Autodesk Inventor part; units mm, degrees
ref_plane "YZ Plane" through (0, 0, 0) normal (1, 0, 0) x (0, 1, 0)
ref_plane "XZ Plane" through (0, 0, 0) normal (0, 1, 0) x (-1, 0, 0)
ref_plane "XY Plane" through (0, 0, 0) normal (0, 0, 1) x (1, 0, 0)
sketch "Sketch1" plane through (0, 0, 0) normal (0, 1, 0) x (-1, 0, 0)
  line L0 (10, -17.5) -> (-10, -17.5)
  line L1 (-10, -17.5) -> (-10, 18.5)
  line L2 (-10, 18.5) -> (10, 18.5)
  line L3 (10, 18.5) -> (10, -17.5)
  point P0 (0, 0)
  dimension "d0" = 20
  dimension "d1" = 36
  dimension "d2" = 17.5
  dimension "d3" = 10
extrude "Plate1" add sketch "Sketch1" along normal blind 1.5
sketch "Sketch2" plane through (-10, 0, -19) normal (0, 0, 1) x (1, 0, 0)
  line L0 (20, 0) -> (0, 0)
  line L1 (0, 0) -> (0, 45.1)
  line L2 (0, 45.1) -> (20, 45.1)
  line L3 (20, 45.1) -> (20, 0)
edge flange "Flange1" height 45.1 angle 90 thickness 1.5 bend radius 0.31 thickness toward (0, 0, 1) relief tear relief width 1.5 relief depth 0.75 edges at (0, 1.5, -17.5) wall of the first edge with corners at (10, 0, -19) (-10, 0, -19) (-10, 45.1, -19) (10, 45.1, -19)
bend "Bend1"
corner "Corner1"
sketch "Sketch3" plane through (10, 0, 20) normal (0, 0, -1) x (-1, 0, 0)
  line L0 (20, 0) -> (0, 0)
  line L1 (0, 0) -> (0, 45.1)
  line L2 (0, 45.1) -> (20, 45.1)
  line L3 (20, 45.1) -> (20, 0)
edge flange "Flange2" height 45.1 angle 90 thickness 1.5 bend radius 0.31 thickness toward (0, 0, -1) relief tear relief width 1.5 relief depth 0.75 edges at (0, 1.5, 18.5) wall of the first edge with corners at (-10, 0, 20) (10, 0, 20) (10, 45.1, 20) (-10, 45.1, 20)
bend "Bend2"
corner "Corner2"
sketch "Sketch4" plane through (-10, 45.1, 20) normal (0, 0, 1) x (1, 0, 0)
  circle A0 centre (10, -10) radius 10
  line L0 (0, 0) -> (20, 0)
  line L1 (0, 0) -> (20, 0)
  line L2 (20, 0) -> (20, -10)
  line L3 (20, -10) -> (0, -10)
  line L4 (0, -10) -> (0, 0)
  line L5 (0, -43.29) -> (0, 0)
  point P0 (10, -45.1)
  point P1 (10, -10)
  point P2 (20, 0)
  point P3 (10, 0)
  point P4 (0, -10)
  point P5 (8.5893, 0)
  point P6 (0, -10)
  dimension "d26" = 20
  dimension "d25" = 10
  dimension "d27" = 10
  dimension "d28" = 10
extrude "Extrusion1" cut sketch "Sketch4" against normal blind 10 contours L4 L0 A0 | A0 L0 L2
sketch "Sketch5" plane through (10, 45.1, -19) normal (0, 0, -1) x (-1, 0, 0)
  arc A0 (20, -10) -> (0, -10) centre (10, -10) ccw
  point P0 (10, -45.1)
hole "Hole1" at (0, 35.1, -19) direction (0, 0, 1) diameter 13.5 depth 1.5
sketch "Sketch6" plane through (10, 45.1, -19) normal (0, 0, -1) x (-1, 0, 0)
  circle A0 centre (10, -10) radius 6.75
  line L0 (0, 0) -> (20, 0)
  line L1 (0, -43.29) -> (0, 0)
  line L2 (24, 0) -> (-4, 0)
  line L3 (-4, 0) -> (-4, -9.9)
  line L4 (-4, -9.9) -> (24, -9.9)
  line L5 (24, -9.9) -> (24, 0)
  point P0 (10, -45.1)
  point P1 (20, 0)
  point P2 (6.005, 0)
  point P3 (13.995, 0)
  dimension "d38" = 9.9
  dimension "d39" = 4
  dimension "d40" = 28
extrude "Extrusion2" cut sketch "Sketch6" against normal blind 10 contours L4 A0 | A0 L4 L1 L0 L2 L5 | L4 L3 L2 L1 picked at (7.8223, -9.3675)
fillet "Fillet1" radius 1 2 edges at (-10, 35.2, -18.25) (10, 35.2, -18.25)
sketch "Sketch7" plane through (-10, 1.81, 20) normal (0, 0, 1) x (1, 0, 0)
  arc A0 (20, 33.29) -> (0, 33.29) centre (10, 33.29) ccw
  point P0 (10, -1.81)
hole "Hole2" at (0, 35.1, 20) direction (0, 0, -1) diameter 5.1 depth 1.5
sketch "Sketch8" plane through (0, 0, 0) normal (0, -1, 0) x (1, 0, 0)
  line L0 (2.55, 18.5) -> (-2.55, 18.5)
  line L1 (-10, 18.5) -> (10, 18.5)
  line L2 (10, 18.5) -> (-10, 18.5)
  line L3 (10, 18.19) -> (-10, 18.19)
  line L4 (-10, -17.19) -> (-10, 18.19)
  line L5 (-10, -17.19) -> (10, -17.19)
  line L6 (10, 18.19) -> (10, -17.19)
  point P0 (0, 0)
  point P1 (7, 9.5)
  point P2 (7, -4.5)
  point P3 (-7, 9.5)
  point P4 (-7, -4.5)
  dimension "d51" = 9
  dimension "d52" = 3
  dimension "d55" = 14
  dimension "d58" = 14
hole "Hole3" at (7, 0, 9.5) at (7, 0, -4.5) at (-7, 0, 9.5) at (-7, 0, -4.5) direction (0, 1, 0) diameter 3 depth 1.5
sketch "Sketch11" plane through (-10, 1.81, -17.5) normal (0, 0, 1) x (1, 0, 0)
  circle A0 centre (18, 26.39) radius 0.7835
  circle A1 centre (2, 26.39) radius 0.7835
  circle A2 centre (17, 13.17) radius 0.7835
  circle A3 centre (3, 13.17) radius 0.7835
  circle A4 centre (10, 5.87) radius 0.7835
  point P0 (10, -1.81)
hole "Hole6" at (-8, 28.2, -17.5) at (-7, 14.98, -17.5) at (0, 7.68, -17.5) at (7, 14.98, -17.5) at (8, 28.2, -17.5) direction (0, 0, -1) diameter 2.1 depth 1.5
sketch "Sketch12" plane through (-10, 1.81, 20) normal (0, 0, 1) x (1, 0, 0)
  line L0 (20, -1.81) -> (0, -1.81)
  circle A0 centre (10, 5.87) radius 1.05
  point P0 (10, -1.81)
hole "Hole7" at (0, 7.68, 20) direction (0, 0, -1) diameter 3 depth 1.5
equation "\"d36\" = Thickness"
equation "\"d49\" = Thickness"
equation "\"d66\" = Thickness"
equation "\"d87\" = Thickness"
equation "\"d94\" = Thickness"
equation "\"d4\" = Thickness"
equation "\"d5\" = BendReliefWidth"
equation "\"d6\" = BendReliefDepth"
equation "\"d7\" = MinimumRemnant"
equation "\"d8\" = TransitionRadius"
equation "\"d11\" = BendRadius"
equation "\"d12\" = CornerReliefSize"
equation "\"d13\" = GapSize"
equation "\"d14\" = JacobiRadiusSize"
equation "\"d15\" = BendReliefWidth"
equation "\"d16\" = BendReliefDepth"
equation "\"d17\" = MinimumRemnant"
equation "\"d18\" = TransitionRadius"
equation "\"d21\" = BendRadius"
equation "\"d22\" = CornerReliefSize"
equation "\"d23\" = GapSize"
equation "\"d24\" = JacobiRadiusSize"
equation "\"BendReliefWidth\" = Thickness"
equation "\"BendReliefDepth\" = 0.5 * Thickness"
equation "\"CornerReliefSize\" = 4 * Thickness"
equation "\"MinimumRemnant\" = 2 * Thickness"
equation "\"TransitionRadius\" = BendRadius"
equation "\"JacobiRadiusSize\" = BendRadius"
equation "\"GapSize\" = Thickness"
properties part number "axis_9_bottom_frame" material "Aluminum 6061-AHC"
CAD build for the part. Positions are in the model's coordinates, mm. A direction names the side the tool comes from. Round coordinates to 2 decimals unless told otherwise and drop trailing zeros. Write each loop counter-clockwise with the first axis right and the second up, starting at its lowest first coordinate (ties: lowest second). Pieces come first, ordered by that corner, then holes.
(1) Probe line 1 along X through (y, z) = (1.05, 9.5); line 2 along Z through (x, y) = (6, 28.5); line 3 along X through (y, z) = (28, -18). List the from-to ranges inside material, lowest first.
(2) Drop flat-ended pins along their axis: P1, Ø5, axis at x = 7, z = -4.5, coming from the +Y side; P2, Ø2.5, axis at x = -8, y = 28.2, coming from the -Z side; P3, Ø2.5, axis at x = 0, y = 7.68, coming from the +Z side; P4, Ø1.6, axis at x = -7.5, z = -18, coming from the +Y side. Give the stop position or say it passes through.
(3) Slice it at A-A, the plane y = 25.5. Write the cut outline in (x, z).
(4) 3-axis set-ups, long thin cutter, end or side, ignore diameter. For faces 1 (the face through (9.699, 34.915, -18.26)), 2 (the face through (0, 1.5, 1)), 3 (the face through (-9.715, 34.899, -18.26)), 4 (the face through (-7.32, 13.98, -18.26)): which of +Z, -Z, +X, -X, +Y, -Y reach the whole face in a straight line?
(5) Mould opens along Y. For faces 5 (the face through (-0.07, 9.18, 19.24)), 6 (the face through (-8.71, 28.974, -18.26)), 7 (the face through (10, 1, 1)), 8 (the face through (0.2, 45.1, 19.3)) say: pulls with the +Y half, pulls with the -Y half, needs draft (parallel to the pull), parting line crosses it, or undercut.
(6) Slice it at C-C, the plane y = 7.68. Write the cut outline in (x, z), and give its area (4 significant figures).
(7) Slice it at D-D, the plane y = 14.98. Write the cut outline in (x, z), and give its area (3 significant figures).
(8) Slice it at B-B, the plane z = 9.5. Write the cut outline in (x, y).
From the geometry:
1. line 1: x = -10 to -8.5, -5.5 to 5.5, 8.5 to 10
1. line 2: z = -19 to -17.5, 18.5 to 20
1. line 3: x = -10 to -9.03, -6.97 to 6.97, 9.03 to 10
2. P1: stops at y = 1.5
2. P2: stops at z = -19
2. P3: stops at z = -17.5
2. P4: stops at y = 35.2
3. outline: (-10, -19) - (10, -19) - (10, -17.5) - (-10, -17.5) - close; (-10, 18.5) - (10, 18.5) - (10, 20) - (-10, 20) - close
4. face 1: -Z, +X, +Y
4. face 2: +X, -X, +Y
4. face 3: -Z, -X, +Y
4. face 4: -Z
5. face 5: undercut
5. face 6: undercut
5. face 7: needs draft
5. face 8: pulls with the +Y half
6. outline: (-10, -19) - (-1.05, -19) - (-1.05, -17.5) - (-10, -17.5) - close; (-10, 18.5) - (-1.5, 18.5) - (-1.5, 20) - (-10, 20) - close; (1.05, -19) - (10, -19) - (10, -17.5) - (1.05, -17.5) - close; (1.5, 18.5) - (10, 18.5) - (10, 20) - (1.5, 20) - close
6. area: 52.35 mm2
7. outline: (-10, -19) - (-8.05, -19) - (-8.05, -17.5) - (-10, -17.5) - close; (-10, 18.5) - (10, 18.5) - (10, 20) - (-10, 20) - close; (-5.95, -19) - (5.95, -19) - (5.95, -17.5) - (-5.95, -17.5) - close; (8.05, -19) - (10, -19) - (10, -17.5) - (8.05, -17.5) - close
7. area: 53.7 mm2
8. outline: (-10, 0) - (-8.5, 0) - (-8.5, 1.5) - (-10, 1.5) - close; (-5.5, 0) - (5.5, 0) - (5.5, 1.5) - (-5.5, 1.5) - close; (8.5, 0) - (10, 0) - (10, 1.5) - (8.5, 1.5) - close
